```python
from build123d import *

# Parameters (mm, degrees)
F1_DEPTH = 3.75
F2_DEPTH = 2.125
F3_SIZE  = 1


# Not quite as in the source:
# - a feature names something its author has since deleted; it is built from what else it names


with BuildPart() as f1:
    # F0 (on Front) → F1 (new body, symmetric)
    with BuildSketch(Plane.XZ):
        Polygon((-15.2139038764, 1.5), (-15.2139038764, 0), (14.7860961236, 0), (14.7860961236, 1.5), (12.7860961236, 1.5), (-13.2139038764, 1.5), align=None)
    extrude(amount=F1_DEPTH, both=True)

    # F0 (on Front) → F2 (join, symmetric)
    with BuildSketch(Plane.XZ):
        with BuildLine():
            Line((-13.2139038764, 3.75), (-13.2139038764, 1.5))
            Line((-13.2139038764, 1.5), (12.7860961236, 1.5))
            Line((12.7860961236, 1.5), (12.7860961236, 3.5))
            ThreePointArc((12.7860961236, 3.5), (12.6093194283, 3.5732233047), (12.5360961236, 3.75))
            Line((12.5360961236, 3.75), (6.9810911579, 3.75))
            Line((6.9810911579, 3.75), (6.5964757732, 5.7126693573))
            Line((6.5964757732, 5.7126693573), (12.2487553674, 7.7255616518))
            Line((12.2487553674, 7.7255616518), (10.9207582075, 13.320105739))
            ThreePointArc((10.9207582075, 13.320105739), (10.6249391085, 13.4870718246), (10.7686600969, 13.794855662))
            Line((10.7686600969, 13.794855662), (9.9194281634, 15.8784355437))
            Line((9.9194281634, 15.8784355437), (12.6975346723, 17.0107447883))
            ThreePointArc((12.6975346723, 17.0107447883), (13.5139207983, 17.8179208397), (13.5204333045, 18.965952665))
            ThreePointArc((13.5204333045, 18.965952665), (12.713257253, 19.782338791), (11.5652254277, 19.7888512971))
            Line((11.5652254277, 19.7888512971), (-18.0679106669, 7.7108860217))
            ThreePointArc((-18.0679106669, 7.7108860217), (-18.8842967929, 6.9037099703), (-18.8908092991, 5.755678145))
            ThreePointArc((-18.8908092991, 5.755678145), (-18.0836332477, 4.939292019), (-16.9356014224, 4.9327795128))
            Line((-16.9356014224, 4.9327795128), (-14.1574949135, 6.0650887574))
            Line((-14.1574949135, 6.0650887574), (-13.2139038764, 3.75))
        make_face()
        with BuildLine():
            ThreePointArc((12.5360961236, 3.75), (12.6093194283, 3.5732233047), (12.7860961236, 3.5))
            Line((12.7860961236, 3.5), (12.7860961236, 3.75))
            Line((12.7860961236, 3.75), (12.5360961236, 3.75))
        make_face()
        with BuildLine():
            Line((12.7860961236, 3.75), (12.7860961236, 3.5))
            ThreePointArc((12.7860961236, 3.5), (12.9628728189, 3.5732233047), (13.0360961236, 3.75))
            ThreePointArc((13.0360961236, 3.75), (12.7860961236, 4), (12.5360961236, 3.75))
            Line((12.5360961236, 3.75), (12.7860961236, 3.75))
        make_face()
        with BuildLine():
            Line((10.8630192006, 13.5633467863), (10.9207582075, 13.320105739))
            ThreePointArc((10.9207582075, 13.320105739), (11.0591502177, 13.4083221943), (11.1130192006, 13.5633467863))
            ThreePointArc((11.1130192006, 13.5633467863), (11.0025007837, 13.7708194061), (10.7686600969, 13.794855662))
            Line((10.7686600969, 13.794855662), (10.8630192006, 13.5633467863))
        make_face()
        with BuildLine():
            ThreePointArc((10.7686600969, 13.794855662), (10.6249391085, 13.4870718246), (10.9207582075, 13.320105739))
            Line((10.9207582075, 13.320105739), (10.8630192006, 13.5633467863))
            Line((10.8630192006, 13.5633467863), (10.7686600969, 13.794855662))
        make_face()
    extrude(amount=F2_DEPTH, both=True)

    # F3
    f3_edges = [f1.edges().sort_by_distance(p)[0] for p in [
        (14.786096, 0, 0),
        (-15.213904, 0, 0),
    ]]
    chamfer(f3_edges, length=F3_SIZE)


solid = f1.part
```
Geometry check sheet. Reference: the model listing, model coordinates, mm. A direction names the side the tool comes from. Coordinates: 2 decimals unless noted, no trailing zeros. Order: outer loops, then holes, each group sorted by start corner. A loop starts at its lowest first (then second) coordinate and runs counter-clockwise, first axis right, second up.
Item 1: Section check C-C (y = 3). Enter the section's corners in (x, z).
Item 2: Depth check by flat-ended pin: pin 1 (1.3 mm diameter, centred on x = 11, y = -0.5, fed in from +Z); pin 2 (1.6 mm diameter, centred on y = 0, z = 2.5, fed in from +X); pin 3 (2 mm diameter, centred on x = 6.5, z = 15.5, fed in from -Y) (3 decimals). Enter the tip coordinate at first touch or a pass-through.
Item 3: Mould release check, pull along Z, two halves, no side actions. Record for faces 1 (the flat face through (-14.707, 0.052, 0.493)), 2 (the flat face through (-13.214, 0, 3)), 3 (the cylindrical face through (-18.903, -0.03, 5.786)), 4 (the flat face through (1, 2.125, 9)): released by +Z, released by -Z, zero draft, split by the parting line, or undercut.
Item 4: Section check A-A (y = -0.25). Enter the section's corners in (x, z), plus the area to 3 significant figures.
Item 5: Section check D-D (z = 11). Enter the section's corners in (x, y) (1 decimal), plus the area to 3 significant figures.
Item 6: Scan lines: line 1 along Y through (x, z) = (-10.5, 2.5) (3 decimals); line 2 along X through (y, z) = (-0.25, 2); line 3 along Z through (x, y) = (-14, -3.5). Record each from-to range of solid material in increasing order.
Item 7: Section check B-B (x = 1). Enter the section's corners in (y, z) (3 decimals).
Item 8: Tool access check on faces 5 (the flat face through (14.293, 0.052, 0.507)), 6 (the flat face through (-3.044, -0.03, 13.834)), 7 (the flat face through (10, 0, 3.75)), 8 (the flat face through (1, -2.125, 9)), 9 (the flat face through (11.594, -0.03, 10.484)). Record the directions out of +Z, -Z, +X, -X, +Y, -Y that give a thin tool (end or side, any length) a straight path to the whole face; none if there is none.
Check sheet entries:
1. outline: (-15.21, 1) - (-14.21, 0) - (13.79, 0) - (14.79, 1) - (14.79, 1.5) - (-15.21, 1.5) - close
2. pin 1: stops at z = 19.82
2. pin 2: stops at x = 12.79
2. pin 3: stops at y = -2.125
3. face 1: released by -Z
3. face 2: undercut
3. face 3: split by the parting line
3. face 4: zero draft
4. outline: (-18.07, 7.71) arc R1.5 ccw to (-16.94, 4.93) - (-14.16, 6.07) - (-13.21, 3.75) - (-13.21, 1.5) - (-15.21, 1.5) - (-15.21, 1) - (-14.21, 0) - (13.79, 0) - (14.79, 1) - (14.79, 1.5) - (12.79, 1.5) - (12.79, 3.5) arc R0.25 ccw (long way) to (12.54, 3.75) - (6.98, 3.75) - (6.6, 5.71) - (12.25, 7.73) - (10.92, 13.32) arc R0.25 ccw (long way) to (10.77, 13.79) - (9.92, 15.88) - (12.7, 17.01) arc R1.5 ccw to (11.57, 19.79) - close
4. area: 382 mm2
5. outline: (-10, -2.1) - (11.5, -2.1) - (11.5, 2.1) - (-10, 2.1) - close
5. area: 91.2 mm2
6. line 1: y = -2.125 to 2.125
6. line 2: x = -13.21 to 12.79
6. line 3: z = 0 to 1.5
7. outline: (-3.75, 0) - (3.75, 0) - (3.75, 1.5) - (2.125, 1.5) - (2.125, 15.483) - (-2.125, 15.483) - (-2.125, 1.5) - (-3.75, 1.5) - close
8. face 5: -Z, +X, +Y, -Y
8. face 6: +Z, -X, +Y, -Y
8. face 7: +Y, -Y
8. face 8: +Z, +X, -X, -Y
8. face 9: +X, +Y, -Y
